Geometry check sheet. Reference: the model listing, model coordinates, mm. A direction names the side the tool comes from. Coordinates: 2 decimals unless noted, no trailing zeros. Write each loop counter-clockwise with the first axis right and the second up, starting at its lowest first coordinate (ties: lowest second). Pieces come first, ordered by that corner, then holes. Notation, with made-up numbers: M -27.5,55.5 L 19.5,55.5 A23 cw 19.5,69.5 Z; hole C -12.75,2.25 d6. An arc over 180 degrees is marked long. Write each question's results on one line, items separated by ' | '.
```python
from build123d import *

# Parameters (mm, degrees)
CROQUIS1_W              = 350
CROQUIS1_H              = 40
SALIENTE_EXTRUIR1_DEPTH = 45
CROQUIS2_W              = 42.2
CROQUIS2_H              = 42.2
CORTAR_EXTRUIR1_DEPTH   = 30
CROQUIS3_R              = 11.125
CORTAR_EXTRUIR2_DEPTH   = 30
CROQUIS4_R              = 11.125
CORTAR_EXTRUIR3_DEPTH   = 186.067555233


with BuildPart() as part:
    # Croquis1 → Saliente-Extruir1 (new body)
    with BuildSketch(Plane(origin=(0, 0, 0), x_dir=(1, 0, 0), z_dir=(0, 1, 0))):
        Rectangle(CROQUIS1_W, CROQUIS1_H)
    extrude(amount=SALIENTE_EXTRUIR1_DEPTH)

    # Croquis2 → Cortar-Extruir1 (cut)
    with BuildSketch(Plane(origin=(0, 0, -20), x_dir=(-1, 0, 0), z_dir=(0, 0, -1))):
        with Locations((-143.9, 21.1)):
            Rectangle(CROQUIS2_W, CROQUIS2_H)
    cortar_extruir1 = extrude(amount=-CORTAR_EXTRUIR1_DEPTH, mode=Mode.SUBTRACT)

    # Croquis3 → Cortar-Extruir2 (cut)
    with BuildSketch(Plane(origin=(0, 0, 10), x_dir=(-1, 0, 0), z_dir=(0, 0, -1))):
        with Locations((-143.9, 21.1)):
            Circle(CROQUIS3_R)
    cortar_extruir2 = extrude(amount=-CORTAR_EXTRUIR2_DEPTH, mode=Mode.SUBTRACT)

    # Simetría1: Cortar-Extruir1, Cortar-Extruir2 across plane
    add(cortar_extruir1.mirror(Plane(origin=(0, 0, 0), x_dir=(0, 0, 1), z_dir=(1, 0, 0))), mode=Mode.SUBTRACT)
    add(cortar_extruir2.mirror(Plane(origin=(0, 0, 0), x_dir=(0, 0, 1), z_dir=(1, 0, 0))), mode=Mode.SUBTRACT)

    # Croquis4 → Cortar-Extruir3 (cut, through all)
    with BuildSketch(Plane.XY.offset(20)):
        Polygon((25, 15), (25, 0), (175, 0), (175, 45), (25, 45), (25, 30), (-25, 30), (-25, 15), align=None)
        with Locations((143.9, 21.1)):
            Circle(CROQUIS4_R, mode=Mode.SUBTRACT)
    extrude(amount=-CORTAR_EXTRUIR3_DEPTH, mode=Mode.SUBTRACT)


solid = part.part
```
Q1. Sectioned sample at A-A on y = 21.1. Record the cut outline in (x, z) (3 decimals), and give its area (3 significant figures).
Geometry check:
outline: M -175,-20 L -165,-20 L -165,10 L -155.025,10 L -155.025,20 L -175,20 Z; M -132.775,10 L -122.8,10 L -122.8,-20 L -25,-20 L -25,20 L -132.775,20 Z | area: 4,510 mm2
Q2. Mould release check, pull along X, two halves, no side actions. Record for faces 1 (the flat face through (-76, 22, 20)), 2 (the flat face through (-165, 21, -5)), 3 (the flat face through (25, 38, 0)): pulls with the +X half, pulls with the -X half, needs draft (parallel to the pull), parting line crosses it, or undercut.
Geometry check:
face 1: needs draft | face 2: undercut | face 3: pulls with the +X half
Q3. Access from +Z, -Z, +X, -X, +Y, -Y to the whole of each face (thin tool, end or side, straight path). Record for faces 4 (the flat face through (0, 15, 0)), 5 (the flat face through (-144, 42.2, -5)), 6 (the flat face through (25, 8, 0)).
Geometry check:
face 4: +Z, -Z, +X | face 5: -Z, -Y | face 6: +Z, -Z, +X, +Y, -Y
Q4. Sectioned sample at C-C on z = 16. Record the cut outline in (x, y) (3 decimals).
Geometry check:
outline: M -175,0 L 25,0 L 25,15 L -25,15 L -25,30 L 25,30 L 25,45 L -175,45 Z; hole C -143.9,21.1 d22.25
Q5. Sectioned sample at B-B on x = -143.9. Record the cut outline in (y, z) (3 decimals).
Geometry check:
outline: M 0,10 L 9.975,10 L 9.975,20 L 0,20 Z; M 32.225,10 L 42.2,10 L 42.2,-20 L 45,-20 L 45,20 L 32.225,20 Z
Q6. Depth check by flat-ended pin: P1, Ø15, axis at x = -134, z = 0.5, coming from the -Y side; P2, Ø24, axis at y = 20.5, z = -1, coming from the +X side; P3, Ø4.5, axis at y = 20, z = 3.5, coming from the +X side; P4, Ø12.5, axis at x = -142, y = 31.5, coming from the -Z side. Enter the tip coordinate at first touch or a pass-through.
Geometry check:
P1: stops at y = 42.2 | P2: stops at x = 25 | P3: stops at x = -25 | P4: stops at z = 10
Q7. Sectioned sample at D-D on y = 4. Record the cut outline in (x, z).
Geometry check:
outline: M -175,-20 L -165,-20 L -165,10 L -122.8,10 L -122.8,-20 L 25,-20 L 25,20 L -175,20 Z
Q8. Scan lines: probe 1 along X at (y, z) = (21, 13); probe 2 along X at (y, z) = (39.5, -1.5); probe 3 along Y at (x, z) = (-143, 17). Record each from-to range of solid material in increasing order.
Geometry check:
probe 1: x = -175 to -155.02, -132.78 to -25 | probe 2: x = -175 to -165, -122.8 to 25 | probe 3: y = 0 to 10.01, 32.19 to 45
